Can you work these out from the model? Positions are in its coordinate system, mm. Face numbers are marked on the shaded views. Give positions to 0.01 mm unless a question says otherwise; leave off trailing zeros. Loops run counter-clockwise (first coordinate to the right, second up) from the corner with the lowest first, then second, coordinate; pieces in that order, holes last. Notation, with made-up numbers: (89, 11.5) - (99, 11.5) arc R20 ccw to (99, 19.5) - close; hole circle Ø2 at (56.5, 56.5). An arc over 180 degrees is marked (long way). Answer as a JSON object with one key per item and string values.
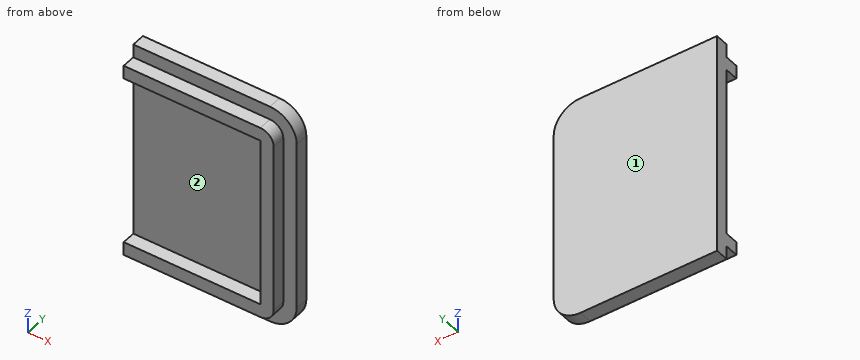
```python
from build123d import *

# Parameters (mm, degrees)
SALIENTE_EXTRUIR1_DEPTH = 5
SALIENTE_EXTRUIR2_DEPTH = 5


with BuildPart() as part:
    # Croquis1 → Saliente-Extruir1 (new body)
    with BuildSketch(Plane(origin=(0, 0, 0), x_dir=(1, 0, 0), z_dir=(0, 1, 0))):
        with BuildLine():
            Line((-30.5, -42.075), (20.5, -42.075))
            ThreePointArc((20.5, -42.075), (27.571067812, -39.146067812), (30.5, -32.075))
            Line((30.5, -32.075), (30.5, 32.075))
            ThreePointArc((30.5, 32.075), (27.571067812, 39.146067812), (20.5, 42.075))
            Line((20.5, 42.075), (-30.5, 42.075))
            Line((-30.5, 42.075), (-30.5, -42.075))
        make_face()
    extrude(amount=SALIENTE_EXTRUIR1_DEPTH)

    # Croquis2 → Saliente-Extruir2 (add)
    with BuildSketch(Plane(origin=(0, 0, 0), x_dir=(1, 0, 0), z_dir=(0, 1, 0))):
        with BuildLine():
            Line((-30.5, -32.075), (20.5, -32.075))
            Line((20.5, -32.075), (20.5, 32.075))
            Line((20.5, 32.075), (-30.5, 32.075))
            Line((-30.5, 32.075), (-30.5, 37.075))
            Line((-30.5, 37.075), (20.5, 37.075))
            ThreePointArc((20.5, 37.075), (24.035533906, 35.610533906), (25.5, 32.075))
            Line((25.5, 32.075), (25.5, -32.075))
            ThreePointArc((25.5, -32.075), (24.035533906, -35.610533906), (20.5, -37.075))
            Line((20.5, -37.075), (-30.5, -37.075))
            Line((-30.5, -37.075), (-30.5, -32.075))
        make_face()
    extrude(amount=-SALIENTE_EXTRUIR2_DEPTH)


solid = part.part
```
1) Imagine slicing it at D-D on x = 23.5. Write out the boundary of the cut face in (y, z) (3 decimals), and give its area (3 significant figures).
Check sheet entries:
{"outline": "(-5, -36.075) - (0, -36.075) - (0, -41.614) - (5, -41.614) - (5, 41.614) - (0, 41.614) - (0, 36.075) - (-5, 36.075) - close", "area": "777 mm2"}
2) Imagine slicing it at A-A on z = -29.5. Write out the boundary of the cut face in (x, y).
Check sheet entries:
{"outline": "(-30.5, 0) - (20.5, 0) - (20.5, -5) - (25.5, -5) - (25.5, 0) - (30.5, 0) - (30.5, 5) - (-30.5, 5) - close"}
3) I need wall thicknesses on L1, parallel to Z at x = 18.5, y = -1.25 (3 decimals); L2, parallel to Y at x = -3, z = 23; L3, parallel to X at y = -2.25, z = 4. Which ranges of each line are inside material? Lowest first, please.
Check sheet entries:
{"L1": "-37.075 to -32.075, 32.075 to 37.075", "L2": "0 to 5", "L3": "20.5 to 25.5"}
4) Imagine slicing it at B-B on x = -20. Write out the boundary of the cut face in (y, z) (3 decimals).
Check sheet entries:
{"outline": "(-5, -37.075) - (0, -37.075) - (0, -42.075) - (5, -42.075) - (5, 42.075) - (0, 42.075) - (0, 37.075) - (-5, 37.075) - (-5, 32.075) - (0, 32.075) - (0, -32.075) - (-5, -32.075) - close"}
5) I'm going to push flat-ended pins straight in: P1, Ø3, axis at y = -0.5, z = -19.5, coming from the +X side; P2, Ø1.5, axis at x = -16.5, y = -2, coming from the -Z side (3 decimals); P3, Ø4, axis at x = 3, y = -2.5, coming from the +Z side (3 decimals); P4, Ø2.5, axis at y = -3.5, z = 14, coming from the -X side. Where does each tip first touch, or does it pass through?
Check sheet entries:
{"P1": "x = 30.5", "P2": "z = -37.075", "P3": "z = 37.075", "P4": "x = 20.5"}
6) If we mould it in two halves opening along Z, with no side actions, what happens to the marked faces 1 and 2? For each: released by +Z, released by -Z, zero draft, split by the parting line, or undercut.
Check sheet entries:
{"face 1": "zero draft", "face 2": "undercut"}
7) Imagine slicing it at C-C on y = -1.25. Write out the boundary of the cut face in (x, z) (3 decimals).
Check sheet entries:
{"outline": "(-30.5, -37.075) - (20.5, -37.075) arc R5 ccw to (25.5, -32.075) - (25.5, 32.075) arc R5 ccw to (20.5, 37.075) - (-30.5, 37.075) - (-30.5, 32.075) - (20.5, 32.075) - (20.5, -32.075) - (-30.5, -32.075) - close"}
